Here's how the part is built. I have some questions about the finished solid (model axes, mm). A direction names the side the tool comes from. Coordinates: 2 decimals unless noted, no trailing zeros.
from build123d import *

# Parameters (mm, degrees)
SKETCH_3_R          = 37.5
EXTRUDE_1_DEPTH     = 2
CUT_EXTRUDE_5_DEPTH = 1.2
SKETCH_4_W          = 5
SKETCH_4_H          = 0.8
CUT_EXTRUDE_6_DEPTH = 54.070707551
SKETCH_5_R          = 2.4
CUT_EXTRUDE_7_DEPTH = 54.069200107


with BuildPart() as part:
    # Sketch 3 → Extrude 1 (new body)
    with BuildSketch(Plane(origin=(0, 0, 0), x_dir=(1, 0, 0), z_dir=(0, 1, 0))):
        with Locations(Location((0, 0, 0), (0, 0, 270))):
            Circle(SKETCH_3_R)
    extrude(amount=EXTRUDE_1_DEPTH)

    # Sketch 1 → Cut-Extrude 5 (cut)
    with BuildSketch(Plane(origin=(0, 0, 0), x_dir=(1, 0, 0), z_dir=(0, 1, 0))):
        Polygon((13.393920133, -32.335783638), (32.335783638, -13.393920133), (32.335783638, 13.393920133), (13.393920133, 32.335783638), (-13.393920133, 32.335783638), (-32.335783638, 13.393920133), (-32.335783638, -13.393920133), (-13.393920133, -32.335783638), align=None)
        Polygon((12.97970657, -31.335783638), (31.335783638, -12.97970657), (31.335783638, 12.97970657), (12.97970657, 31.335783638), (-12.97970657, 31.335783638), (-31.335783638, 12.97970657), (-31.335783638, -12.97970657), (-12.97970657, -31.335783638), align=None, mode=Mode.SUBTRACT)
        Polygon((11.671844687, -28.178325742), (28.178325742, -11.671844687), (28.178325742, 11.671844687), (11.671844687, 28.178325742), (-11.671844687, 28.178325742), (-28.178325742, 11.671844687), (-28.178325742, -11.671844687), (-11.671844687, -28.178325742), align=None)
        Polygon((11.257631125, -27.178325742), (27.178325742, -11.257631125), (27.178325742, 11.257631125), (11.257631125, 27.178325742), (-11.257631125, 27.178325742), (-27.178325742, 11.257631125), (-27.178325742, -11.257631125), (-11.257631125, -27.178325742), align=None, mode=Mode.SUBTRACT)
        Polygon((-9.758427525, -23.558928079), (9.758427525, -23.558928079), (23.558928079, -9.758427525), (23.558928079, 9.758427525), (9.758427525, 23.558928079), (-9.758427525, 23.558928079), (-23.558928079, 9.758427525), (-23.558928079, -9.758427525), align=None)
        Polygon((-9.344213963, -22.558928079), (9.344213963, -22.558928079), (22.558928079, -9.344213963), (22.558928079, 9.344213963), (9.344213963, 22.558928079), (-9.344213963, 22.558928079), (-22.558928079, 9.344213963), (-22.558928079, -9.344213963), align=None, mode=Mode.SUBTRACT)
        Polygon((7.749339505, -18.708560533), (18.708560533, -7.749339505), (18.708560533, 7.749339505), (7.749339505, 18.708560533), (-7.749339505, 18.708560533), (-18.708560533, 7.749339505), (-18.708560533, -7.749339505), (-7.749339505, -18.708560533), align=None)
        Polygon((7.335125943, -17.708560533), (17.708560533, -7.335125943), (17.708560533, 7.335125943), (7.335125943, 17.708560533), (-7.335125943, 17.708560533), (-17.708560533, 7.335125943), (-17.708560533, -7.335125943), (-7.335125943, -17.708560533), align=None, mode=Mode.SUBTRACT)
        Polygon((-5.931593202, 14.320132754), (-14.320132754, 5.931593202), (-14.320132754, -5.931593202), (-5.931593202, -14.320132754), (5.931593202, -14.320132754), (14.320132754, -5.931593202), (14.320132754, 5.931593202), (5.931593202, 14.320132754), align=None)
        Polygon((-5.517379639, 13.320132754), (-13.320132754, 5.517379639), (-13.320132754, -5.517379639), (-5.517379639, -13.320132754), (5.517379639, -13.320132754), (13.320132754, -5.517379639), (13.320132754, 5.517379639), (5.517379639, 13.320132754), align=None, mode=Mode.SUBTRACT)
    extrude(amount=CUT_EXTRUDE_5_DEPTH, mode=Mode.SUBTRACT)

    # Sketch 4 → Cut-Extrude 6 (cut, through all)
    with BuildSketch(Plane(origin=(0, 2, 0), x_dir=(1, 0, 0), z_dir=(0, 1, 0))):
        with Locations((-35, 0)):
            Rectangle(SKETCH_4_W, SKETCH_4_H)
        with Locations((35, 0)):
            Rectangle(SKETCH_4_W, SKETCH_4_H)
    extrude(amount=-CUT_EXTRUDE_6_DEPTH, mode=Mode.SUBTRACT)

    # Sketch 5 → Cut-Extrude 7 (cut, through all)
    with BuildSketch(Plane(origin=(0, 2, 0), x_dir=(1, 0, 0), z_dir=(0, 1, 0))):
        with Locations(Location((0, 0, 0), (0, 0, 270))):
            Circle(SKETCH_5_R)
    extrude(amount=-CUT_EXTRUDE_7_DEPTH, mode=Mode.SUBTRACT)


solid = part.part
1. I want a section at A-A (y = 0.75). State how many separate pieces and enclosed holes the cut face has, then the cut area to 3 significant figures.
2. For pin 1 Ø0.6 at (x, y) = (4, 0.5) entering from +Z; pin 2 Ø1 at (x, y) = (34, 1.5) entering from +Z; pin 3 Ø0.6 at (y, z) = (0.5, -1) entering from -X, each with a flat end and sliding along its axis, tell me the tip position at first contact or that it passes through.
3. If I drill on line 1 (X direction, y = 1.4, z = 0); line 2 (Y direction, x = -32, z = -2.5); line 3 (Z direction, x = -19, y = 1.35), over which ranges is the centre line in solid material (lowest first)?
4. Thinking about a two-plate mould opening in Z: for faces 1 (the face through (19.81, 0.59, 20.04)), 2 (the face through (-25, 0, 22)), 3 (the face through (-0.82, 0.99, 37.49)), 4 (the face through (-10.07, 0.59, -10.18)), which applies, pulls with the +Z half, pulls with the -Z half, needs draft (parallel to the pull), parting line crosses it, or undercut?
5. On a 3-axis mill with a long thin cutter (end or side, diameter ignored), from which of +Z, -Z, +X, -X, +Y, -Y can I reach the whole of each face in a straight line? I mean faces 5 (the face through (35, 1, -0.4)), 6 (the face through (22.286, 0.592, -22.029)), 7 (the face through (-9, 0, 12)). Say none if no direction works.
Response values:
1. separate pieces: 6
1. enclosed holes: 6
1. area: 3,630 mm2
2. pin 1: stops at z = 37.32
2. pin 2: stops at z = 16.85
2. pin 3: stops at x = -37.49
3. line 1: x = -32.5 to -2.4, 2.4 to 32.5
3. line 2: y = 1.2 to 2
3. line 3: z = -32.33 to 32.33
4. face 1: undercut
4. face 2: needs draft
4. face 3: pulls with the +Z half
4. face 4: undercut
5. face 5: +X, +Y, -Y
5. face 6: -Y
5. face 7: +Z, -Z, +X, -X, -Y
